Check sheet for the modelled part. Datum: model origin and axes. Units: mm. A direction names the side the tool comes from. Round coordinates to 2 decimals unless told otherwise and drop trailing zeros. Order: outer loops, then holes, each group sorted by start corner. A loop starts at its lowest first (then second) coordinate and runs counter-clockwise, first axis right, second up. Notation, with made-up numbers: (-3.75, 47.25) -> (1.25, 47.25) arc R17 cw to (1.25, 80.25) -> close; hole circle Ø7 at (-25.75, -8.75). An arc over 180 degrees is marked (long way). Answer in a Markdown table with one row per item.
Autodesk Inventor part; units mm, degrees
ref_plane "YZ Plane" through (0, 0, 0) normal (1, 0, 0) x (0, 1, 0)
ref_plane "XZ Plane" through (0, 0, 0) normal (0, 1, 0) x (-1, 0, 0)
ref_plane "XY Plane" through (0, 0, 0) normal (0, 0, 1) x (1, 0, 0)
sketch "Sketch1" plane through (0, 0, 0) normal (0, 0, 1) x (1, 0, 0)
  line L0 (-2, -20) -> (-2, 20)
  line L1 (-2, 20) -> (2, 20)
  line L2 (2, 20) -> (2, -20)
  line L3 (2, -20) -> (-2, -20)
  line L4 (-2, -20) -> (2, 20) construction
  line L5 (-2, 20) -> (2, -20) construction
  line L6 (0, -20) -> (0, -19.6)
  line L7 (0, -20) -> (1.6, -20)
  line L8 (0, -20) -> (-1.6, -20)
  line L9 (-1.6, -20) -> (-2, -19.6)
  line L10 (0, 22.999163) -> (0, 17.000837)
  line L11 (0, 20) -> (0, 24)
  line L12 (0, 24) -> (3.5, 24)
  line L13 (0, 20) -> (3.5, 20)
  line L14 (3.5, 20) -> (3.5, 24)
  line L15 (0, 24) -> (-3.5, 24)
  line L16 (-3.5, 24) -> (-3.5, 20)
  line L17 (-3.5, 20) -> (0, 20)
  line L18 (0, 24) -> (3.1, 24)
  line L19 (0, 24) -> (0, 23.6)
  line L20 (3.1, 24) -> (3.5, 23.6)
  line L21 (0, 24) -> (-3.1, 24)
  line L22 (1.6, -20) -> (2, -19.6)
  line L23 (0, 20) -> (0, -20.824074)
  line L24 (0, -20) -> (0, 20)
  point P0 (0, 0)
  dimension "d0" = 40
  dimension "d1" = 4
  dimension "d2" = 0.4
  dimension "d3" = 1.6
  dimension "d4" = 1.6
  dimension "d5" = 4
  dimension "d6" = 3.5
  dimension "d7" = 3.5
  dimension "d8" = 3.1
  dimension "d9" = 0.4
  dimension "d10" = 3.1
revolve "Revolution1" add sketch "Sketch1" angle 360 about axis through (0, -20, 0) along (0, 1, 0) contours L6 L23 L10 L1 L2 L22 L3 | L10 L11 L12 L20 L14 L13 L1
sketch "Sketch2" plane through (0, 24, 0) normal (0, 1, 0) x (1, 0, 0)
  line L0 (-2.8, -0.625) -> (2.8, -0.625)
  line L1 (2.8, -0.625) -> (2.8, 0.625)
  line L2 (2.8, 0.625) -> (-2.8, 0.625)
  line L3 (-2.8, 0.625) -> (-2.8, -0.625)
  line L4 (-2.8, -0.625) -> (2.8, 0.625) construction
  line L5 (2.8, -0.625) -> (-2.8, 0.625) construction
  line L6 (-0.625, -2.8) -> (-0.625, 2.8)
  line L7 (-0.625, 2.8) -> (0.625, 2.8)
  line L8 (0.625, 2.8) -> (0.625, -2.8)
  line L9 (0.625, -2.8) -> (-0.625, -2.8)
  circle A0 centre (0, 0) radius 2
  line L10 (-0.625, -2.8) -> (0.625, 2.8) construction
  line L11 (-0.625, 2.8) -> (0.625, -2.8) construction
  dimension "d12" = 5.6
  dimension "d13" = 1.25
  dimension "d14" = 5.6
  dimension "d15" = 1.25
sketch "Sketch2 outline for Extrusion1" plane through (0, 24, 0) normal (0, 1, 0) x (1, 0, 0)
  line L0 (-0.625, -2.8) -> (-0.625, -0.625)
  line L1 (0.625, -2.8) -> (-0.625, -2.8)
  line L2 (0.625, -0.625) -> (0.625, -2.8)
  line L3 (0.625, -0.625) -> (2.8, -0.625)
  line L4 (2.8, -0.625) -> (2.8, 0.625)
  line L5 (2.8, 0.625) -> (0.625, 0.625)
  line L6 (0.625, 2.8) -> (0.625, 0.625)
  line L7 (-0.625, 2.8) -> (0.625, 2.8)
  line L8 (-0.625, 0.625) -> (-0.625, 2.8)
  line L9 (-0.625, 0.625) -> (-2.8, 0.625)
  line L10 (-2.8, 0.625) -> (-2.8, -0.625)
  line L11 (-2.8, -0.625) -> (-0.625, -0.625)
extrude "Extrusion1" cut sketch "Sketch2 outline for Extrusion1" against normal blind 2.5 draft -10
properties part number "Screws" material "Steel"
(1) Depth check by flat-ended pin: pin 1 Ø1 at (x, y) = (2, -1) entering from -Z; pin 2 Ø2 at (x, z) = (2.5, -2.5) entering from -Y. Enter the tip coordinate at first touch or a pass-through.
Solutions:
| item | result |
|---|---|
| pin 1 | z = -1.32 |
| pin 2 | y = 20 |
(2) Draft check along X on faces 4 (the cylindrical face through (3.233, 21.825, 1.341)), 5 (the flat face through (1.47, 22.77, 0.41)), 6 (the flat face through (2, 20, 2)). Enter one of: pulls with the +X half, pulls with the -X half, needs draft (parallel to the pull), parting line crosses it, or undercut.
Solutions:
| item | result |
|---|---|
| face 4 | parting line crosses it |
| face 5 | undercut |
| face 6 | needs draft |
(3) Section check A-A on y = -16. Record the boundary of the cut face in (x, z), plus the area to 3 significant figures.
Solutions:
| item | result |
|---|---|
| outline | circle Ø4 at (0, 0) |
| area | 12.6 mm^2 |
(4) Scan lines: probe 1 along Y at (x, z) = (-2, -2); probe 2 along X at (y, z) = (5, 0); probe 3 along Z at (x, y) = (-1.25, 2). Record each from-to range of solid material in increasing order. Write a range as from..to.
Solutions:
| item | result |
|---|---|
| probe 1 | 20..24 |
| probe 2 | -2..2 |
| probe 3 | -1.56..1.56 |
(5) Tool access check on faces 1 (the cylindrical face through (0, 0, -2)), 2 (the flat face through (-1.47, 22.77, -0.41)), 3 (the flat face through (0, -20, 0)). Record the directions out of +Z, -Z, +X, -X, +Y, -Y that give a thin tool (end or side, any length) a straight path to the whole face; none if there is none.
Solutions:
| item | result |
|---|---|
| face 1 | -Y |
| face 2 | +Y |
| face 3 | +Z, -Z, +X, -X, -Y |
